from build123d import *

# Parameters (mm, degrees)
F0_W     = 57.15
F0_H     = 38.1
F1_DEPTH = 25.4
F3_DEPTH = 25.4


with BuildPart() as f1:
    # F0 (on Front) → F1 (new body)
    with BuildSketch(Plane.XZ):
        with Locations((-28.575, 19.05)):
            Rectangle(F0_W, F0_H)
    extrude(amount=F1_DEPTH)

    # F2 (on face) → F3 (cut)
    with BuildSketch(Plane.XZ.offset(25.4)):
        with BuildLine():
            Line((0, 38.1), (-20.702738, 38.1))
            ThreePointArc((-20.702738, 38.1), (-14.283178, 24.302075), (0, 19.05))
            Line((0, 19.05), (0, 38.1))
        make_face()
        with BuildLine():
            ThreePointArc((-57.15, 31.297673), (-54.878227, 35.924092), (-50.205953, 38.1))
            Line((-50.205953, 38.1), (-57.15, 38.1))
            Line((-57.15, 38.1), (-57.15, 31.297673))
        make_face()
    extrude(amount=-F3_DEPTH, mode=Mode.SUBTRACT)


solid = f1.part
Here's how the part is built. I have some questions about the finished solid (model axes, mm). Give positions to 0.01 mm unless a question says otherwise; leave off trailing zeros. Order: outer loops, then holes, each group sorted by start corner. A loop starts at its lowest first (then second) coordinate and runs counter-clockwise, first axis right, second up. Notation, with made-up numbers: (27.5, 88) -> (83.5, 88) arc R10 cw to (83.5, 106) -> close; hole circle Ø1 at (-8.75, 9). An arc over 180 degrees is marked (long way). Use a Markdown table: item, result. Add a question column.
Item 1: Imagine slicing it at A-A on y = -13.75. Please give me the cut outline in (x, z).
Item 2: Imagine slicing it at C-C on x = -14. Please give me the cut outline in (y, z), plus the area to 3 significant figures.
Item 3: Imagine slicing it at B-B on z = 30. Please give me the cut outline in (x, y), plus the area to 3 significant figures.
Item 4: I need wall thicknesses on line 1 (X direction, y = -7.5, z = 31); line 2 (Z direction, x = -5, y = -7.25); line 3 (X direction, y = -15.75, z = 32). Which ranges of each line are inside material? Lowest first, please.
Item 5: Will this pin go through, and if not, where does the flat tip stop? pin 1 (1 mm diameter, centred on x = -10, z = 6.5, fed in from +Y).
Data:
| question | item | result |
|---|---|---|
| 1 | outline | (-57.15, 0) -> (0, 0) -> (0, 19.05) arc R19.94 cw to (-20.7, 38.1) -> (-50.21, 38.1) arc R7.74 ccw to (-57.15, 31.3) -> close |
| 2 | outline | (-25.4, 0) -> (0, 0) -> (0, 24.05) -> (-25.4, 24.05) -> close |
| 2 | area | 611 mm² |
| 3 | outline | (-57.15, -25.4) -> (-18.59, -25.4) -> (-18.59, 0) -> (-57.15, 0) -> close |
| 3 | area | 979 mm² |
| 4 | line 1 | x = -57.15 to -19.06 |
| 4 | line 2 | z = 0 to 19.49 |
| 4 | line 3 | x = -57.03 to -19.46 |
| 5 | pin 1 | stops at y = 0 |
